Can you work these out from the model? Positions are in its coordinate system, mm. A direction names the side the tool comes from. Coordinates: 2 decimals unless noted, no trailing zeros. Write each loop counter-clockwise with the first axis right and the second up, starting at its lowest first coordinate (ties: lowest second). Pieces come first, ordered by that corner, then holes. Notation, with made-up numbers: (53.5, -12) -> (111.5, -12) arc R35 ccw to (111.5, 21) -> close; hole circle Ø5 at (77, 74). An arc over 180 degrees is marked (long way). Use one line per item in the form item = value.
```python
from build123d import *

# Parameters (mm, degrees)
SKETCH1_W                                            = 254
SKETCH1_H                                            = 139.7
BOSS_EXTRUDE1_DEPTH                                  = 19.05
FILLET1_R                                            = 20
SKETCH2_W                                            = 254
SKETCH2_H                                            = 3.05
CUT_EXTRUDE1_DEPTH                                   = 190.757720528
SKETCH8_W                                            = 40
SKETCH8_H                                            = 139.7
CUT_EXTRUDE2_DEPTH                                   = 12
M12_TAPPED_HOLE2_D                                   = 10.2
M12_TAPPED_HOLE2_DEPTH                               = 43.99
M12_TAPPED_HOLE2_TIP                                 = 3.064389157
M12_CLEARANCE_HOLE1_D                                = 13.5
CBORE_FOR_M12_HEX_SOCKET_HEAD_CAP_SCREW1_D           = 13.5
CBORE_FOR_M12_HEX_SOCKET_HEAD_CAP_SCREW1_CBORE_D     = 20
CBORE_FOR_M12_HEX_SOCKET_HEAD_CAP_SCREW1_CBORE_DEPTH = 13
CUT_EXTRUDE3_DEPTH                                   = 5.08
FILLET2_R                                            = 0.79375
FILLET3_R                                            = 1.5875


with BuildPart() as part:
    # Sketch1 → Boss-Extrude1 (new, symmetric)
    with BuildSketch(Plane(origin=(0, 0, 0), x_dir=(1, 0, 0), z_dir=(0, 1, 0))):
        Rectangle(SKETCH1_W, SKETCH1_H)
    extrude(amount=BOSS_EXTRUDE1_DEPTH, both=True)

    # Fillet1
    fillet1_edges = [part.edges().sort_by_distance(p)[0] for p in [
        (-127, 0, -69.85),
        (127, 0, -69.85),
        (127, 0, 69.85),
        (-127, 0, 69.85),
    ]]
    fillet(fillet1_edges, radius=FILLET1_R)

    # Sketch2 → Cut-Extrude1 (cut, through all)
    with BuildSketch(Plane.XY.offset(69.85)):
        with Locations((0, 17.525)):
            Rectangle(SKETCH2_W, SKETCH2_H)
        with Locations((0, -17.525)):
            Rectangle(SKETCH2_W, SKETCH2_H)
    extrude(amount=-CUT_EXTRUDE1_DEPTH, mode=Mode.SUBTRACT)

    # Sketch8 → Cut-Extrude2 (cut)
    with BuildSketch(Plane(origin=(0, 16, 0), x_dir=(1, 0, 0), z_dir=(0, 1, 0))):
        with Locations((-107, 0)):
            Rectangle(SKETCH8_W, SKETCH8_H)
        with Locations((107, 0)):
            Rectangle(SKETCH8_W, SKETCH8_H)
    extrude(amount=-CUT_EXTRUDE2_DEPTH, mode=Mode.SUBTRACT)

    # M12 Tapped Hole2
    with Locations(Plane(origin=(0, 16, 0), x_dir=(-1, 0, 0), z_dir=(0, 1, 0))):
        with Locations((-12, 45), (-12, -45), (-44, -45), (-44, 45)):
            Hole(M12_TAPPED_HOLE2_D / 2, depth=M12_TAPPED_HOLE2_DEPTH)
            with Locations((0, 0, -(M12_TAPPED_HOLE2_DEPTH + M12_TAPPED_HOLE2_TIP / 2))):  # 118° drill point
                Cone(0, M12_TAPPED_HOLE2_D / 2, M12_TAPPED_HOLE2_TIP, mode=Mode.SUBTRACT)

    # M12 Clearance Hole1 (through all)
    with Locations(Plane(origin=(0, 4, 0), x_dir=(1, 0, 0), z_dir=(0, 1, 0))):
        with Locations((-105, 31), (-105, -31), (105, 31), (105, -31)):
            Hole(M12_CLEARANCE_HOLE1_D / 2)

    # CBORE for M12 Hex Socket Head Cap Screw1 (through all)
    with Locations(Plane.XZ.offset(16)):
        with Locations((-36, -31), (-68, 31), (-36, 31), (-68, -31)):
            CounterBoreHole(CBORE_FOR_M12_HEX_SOCKET_HEAD_CAP_SCREW1_D / 2, CBORE_FOR_M12_HEX_SOCKET_HEAD_CAP_SCREW1_CBORE_D / 2, CBORE_FOR_M12_HEX_SOCKET_HEAD_CAP_SCREW1_CBORE_DEPTH)

    # Sketch11 → Cut-Extrude3 (cut)
    with BuildSketch(Plane(origin=(0, 16, 0), x_dir=(1, 0, 0), z_dir=(0, 1, 0))):
        with BuildLine():
            Line((-46, 22.5), (-46, -22.5))
            ThreePointArc((-46, -22.5), (-52, -28.5), (-58, -22.5))
            Line((-58, -22.5), (-58, 22.5))
            ThreePointArc((-58, 22.5), (-52, 28.5), (-46, 22.5))
        make_face()
    extrude(amount=-CUT_EXTRUDE3_DEPTH, mode=Mode.SUBTRACT)

    # Fillet2
    fillet2_edges = [part.edges().sort_by_distance(p)[0] for p in [
        (-52, 10.92, -28.5),
        (-46, 10.92, 0),
        (-52, 10.92, 28.5),
        (-58, 10.92, 0),
    ]]
    fillet(fillet2_edges, radius=FILLET2_R)

    # Fillet3
    fillet3_edges = [part.edges().sort_by_distance(p)[0] for p in [
        (-87, 4, 0),
        (87, 4, 0),
    ]]
    fillet(fillet3_edges, radius=FILLET3_R)


solid = part.part
```
Q1. Will these pins go through, and if not, where does the flat tip stop? pin 1 (15.5 mm diameter, centred on x = -36, z = 31, fed in from -Y); pin 2 (3.5 mm diameter, centred on y = 14, z = 6, fed in from -X); pin 3 (17.5 mm diameter, centred on x = -105, z = -31, fed in from +Y).
Return value:
pin_1 = -3
pin_2 = -87
pin_3 = 4
Q2. Thinking about a two-plate mould opening in Z: for faces 1 (the flat face through (108, 4, -1)), 2 (the cylindrical face through (121.297, -6.14, -63.836)), 3 (the cylindrical face through (39.95, -0.22, -48.1)), 4 (the cylindrical face through (16.711, -0.224, -46.953)), which applies, released by +Z, released by -Z, zero draft, split by the parting line, or undercut?
Return value:
face_1 = zero draft
face_2 = released by -Z
face_3 = undercut
face_4 = undercut
Q3. Suppose I cut it at C-C (x = -68). Write out the boundary of the cut face in (y, z), then the cut area to 3 significant figures.
Return value:
outline = (-16, -69.85) -> (16, -69.85) -> (16, -37.75) -> (-3, -37.75) -> (-3, -41) -> (-16, -41) -> close; (-16, -21) -> (-3, -21) -> (-3, -24.25) -> (16, -24.25) -> (16, 24.25) -> (-3, 24.25) -> (-3, 21) -> (-16, 21) -> close; (-16, 41) -> (-3, 41) -> (-3, 37.75) -> (16, 37.75) -> (16, 69.85) -> (-16, 69.85) -> close
area = 3,440 mm2
Q4. For faces 5 (the cylindrical face through (-71.63, 6.63, -25.31)), 6 (the cylindrical face through (-76, -10, 25)), 7 (the cylindrical face through (-52.1, 13.9, -28.5)), which set-ups out of +Z, -Z, +X, -X, +Y, -Y let a thin tool reach every point of the face, with its end or its side?
Return value:
face_5 = +Y, -Y
face_6 = -Y
face_7 = +Y
Q5. If I drill on line 1 (Z direction, x = 105, y = -5.75); line 2 (Z direction, x = 44, y = -8.5); line 3 (X direction, y = 3.5, z = 48.5), over which ranges is the centre line in solid material (lowest first)? Write a range as from..to.
Return value:
line_1 = -69.85..-37.75, -24.25..24.25, 37.75..69.85
line_2 = -69.85..-50.1, -39.9..39.9, 50.1..69.85
line_3 = -127..8.29, 15.71..40.29, 47.71..127
Q6. Suppose I cut it at A-A (z = -31). Give the number of separate pieces and of enclosed holes in the cut face, then the cut area to 3 significant figures.
Return value:
separate_pieces = 5
enclosed_holes = 0
area = 5,600 mm2
Q7. Suppose I cut it at D-D (z = 11). Write out the boundary of the cut face in (x, y) (1 decimal).
Return value:
outline = (-127, -16) -> (127, -16) -> (127, 4) -> (88.6, 4) arc R1.6 cw to (87, 5.6) -> (87, 16) -> (-46, 16) -> (-46, 11.7) arc R0.8 cw to (-46.8, 10.9) -> (-57.2, 10.9) arc R0.8 cw to (-58, 11.7) -> (-58, 16) -> (-87, 16) -> (-87, 5.6) arc R1.6 cw to (-88.6, 4) -> (-127, 4) -> close
